from build123d import *

# Parameters (mm, degrees)
SKETCH1_R           = 1.200027231
SKETCH1_R_2         = 1.087684018
BOSS_EXTRUDE1_DEPTH = 2.5
BOSS_EXTRUDE2_DEPTH = 9.3
SKETCH3_W           = 40
SKETCH3_H           = 20
BOSS_EXTRUDE3_DEPTH = 36


with BuildPart() as part:
    # Sketch1 → Boss-Extrude1 (new body)
    with BuildSketch(Plane(origin=(0, 0, 0), x_dir=(1, 0, 0), z_dir=(0, 1, 0))):
        with BuildLine():
            Line((1.2, 0), (52.8, 0))
            ThreePointArc((52.8, 0), (53.648528137, 0.351471863), (54, 1.2))
            Line((54, 1.2), (54, 18.8))
            ThreePointArc((54, 18.8), (53.648528137, 19.648528137), (52.8, 20))
            Line((52.8, 20), (1.2, 20))
            ThreePointArc((1.2, 20), (0.351471863, 19.648528137), (0, 18.8))
            Line((0, 18.8), (0, 1.2))
            ThreePointArc((0, 1.2), (0.351471863, 0.351471863), (1.2, 0))
        make_face()
        with Locations(Location((2.75, 16.159014692, 0), (0, 0, 270))):
            Circle(SKETCH1_R, mode=Mode.SUBTRACT)
        with Locations(Location((51.25, 16.159014692, 0), (0, 0, 270))):
            Circle(SKETCH1_R_2, mode=Mode.SUBTRACT)
        with Locations(Location((51.25, 3.840985308, 0), (0, 0, 90))):
            Circle(SKETCH1_R_2, mode=Mode.SUBTRACT)
        with Locations(Location((2.75, 3.840985308, 0), (0, 0, 90))):
            Circle(SKETCH1_R, mode=Mode.SUBTRACT)
    extrude(amount=BOSS_EXTRUDE1_DEPTH)

    # Sketch2 → Boss-Extrude2 (add)
    with BuildSketch(Plane(origin=(0, 2.5, 0), x_dir=(1, 0, 0), z_dir=(0, 1, 0))):
        with BuildLine():
            Line((8.2, 20), (45.8, 20))
            ThreePointArc((45.8, 20), (46.648528137, 19.648528137), (47, 18.8))
            Line((47, 18.8), (47, 1.2))
            ThreePointArc((47, 1.2), (46.648528137, 0.351471863), (45.8, 0))
            Line((45.8, 0), (8.2, 0))
            ThreePointArc((8.2, 0), (7.351471863, 0.351471863), (7, 1.2))
            Line((7, 1.2), (7, 18.8))
            ThreePointArc((7, 18.8), (7.351471863, 19.648528137), (8.2, 20))
        make_face()
    extrude(amount=BOSS_EXTRUDE2_DEPTH)

    # Sketch3 → Boss-Extrude3 (add)
    with BuildSketch(Plane.XZ):
        with Locations((27, -10)):
            Rectangle(SKETCH3_W, SKETCH3_H)
    extrude(amount=BOSS_EXTRUDE3_DEPTH)


solid = part.part
Could you check a few things on this model? Use its own coordinates, in mm. A direction names the side the tool comes from. Round coordinates to 2 decimals unless told otherwise and drop trailing zeros. Write each loop counter-clockwise with the first axis right and the second up, starting at its lowest first coordinate (ties: lowest second). Pieces come first, ordered by that corner, then holes. Notation, with made-up numbers: (29, 81) -> (59, 81) arc R32 ccw to (59, 115) -> close; hole circle Ø1 at (-39.5, 38.5). An arc over 180 degrees is marked (long way). Use a Markdown table: item, result.
1. We'd pull the mould along X, two halves only. Please class faces 4 (the face through (7.342, 7.085, -19.639)), 5 (the face through (46.639, 7.085, -19.658)), 6 (the face through (52.312, 1.232, -3.605)): +X half, -X half, draft (parallel to the pull), parting line (faces both ways), or undercut.
Answer key:
| item | result |
|---|---|
| face 4 | -X half |
| face 5 | +X half |
| face 6 | undercut |
2. If we section it at D-D (x = 51.25): List the corners of the cut face in (y, z) for me.
Answer key:
| item | result |
|---|---|
| outline | (0, -20) -> (2.5, -20) -> (2.5, -17.25) -> (0, -17.25) -> close; (0, -15.07) -> (2.5, -15.07) -> (2.5, -4.93) -> (0, -4.93) -> close; (0, -2.75) -> (2.5, -2.75) -> (2.5, 0) -> (0, 0) -> close |
3. If we section it at C-C (y = -3.5): List the corners of the cut face in (x, z) for me, then the cut area to 3 significant figures.
Answer key:
| item | result |
|---|---|
| outline | (7, -20) -> (47, -20) -> (47, 0) -> (7, 0) -> close |
| area | 800 mm^2 |
4. If we section it at A-A (x = 2.75): List the corners of the cut face in (y, z) for me.
Answer key:
| item | result |
|---|---|
| outline | (0, -20) -> (2.5, -20) -> (2.5, -17.36) -> (0, -17.36) -> close; (0, -14.96) -> (2.5, -14.96) -> (2.5, -5.04) -> (0, -5.04) -> close; (0, -2.64) -> (2.5, -2.64) -> (2.5, 0) -> (0, 0) -> close |
5. Please list where these lines run through material, in increasing order: probe 1 along X at (y, z) = (-8, -12.25); probe 2 along Y at (x, z) = (50, -4.75).
Answer key:
| item | result |
|---|---|
| probe 1 | x = 7 to 47 |
| probe 2 | y = 0 to 2.5 |
6. If we section it at B-B (z = -2): List the corners of the cut face in (x, y) for me.
Answer key:
| item | result |
|---|---|
| outline | (0, 0) -> (7, 0) -> (7, -36) -> (47, -36) -> (47, 0) -> (54, 0) -> (54, 2.5) -> (47, 2.5) -> (47, 11.8) -> (7, 11.8) -> (7, 2.5) -> (0, 2.5) -> close |
7. For pin 1 Ø2 at (x, z) = (2.75, -3.84) entering from +Y; pin 2 Ø12 at (y, z) = (-21.5, -12) entering from +X; pin 3 Ø4 at (x, z) = (2.75, -16.16) entering from -Y; pin 4 Ø6.5 at (x, z) = (48.5, -9.5) entering from +Y, each with a flat end and sliding along its axis, tell me the tip position at first contact or that it passes through.
Answer key:
| item | result |
|---|---|
| pin 1 | passes through |
| pin 2 | stops at x = 47 |
| pin 3 | stops at y = 0 |
| pin 4 | stops at y = 11.8 |
8. Which directions (+Z, -Z, +X, -X, +Y, -Y) give clear straight access to the entire face, cutting with the end or side of a thin tool? Please do faces 1 (the face through (46.658, 7.085, -0.361)), 2 (the face through (7.361, 7.085, -0.342)), 3 (the face through (50, 0, -10)).
Answer key:
| item | result |
|---|---|
| face 1 | +Z, +X, +Y |
| face 2 | +Z, -X, +Y |
| face 3 | +Z, -Z, +X, -Y |
